Design review of the part built by this model. Coordinates are the model's own, in mm. Coordinates: 2 decimals unless noted, no trailing zeros. Answer as a JSON object with one key per item and string values.
from build123d import *

# Parameters (mm, degrees)
SWEEP1_PROFILE_R     = 13.49375
CUT_SWEEP1_PROFILE_R = 9.525


with BuildPart() as part:
    # Sweep1: sweep along a curve in space
    with BuildLine() as sweep1_path:
        Line((144.16623583, 29.78638886, -53.357198813), (145.299475263, 25.359683675, -34.863347144))
        add(Edge.make_bspline(
            [(145.299475263, 25.359683675, -34.863347144), (146.690863379, 19.924587782, -12.156649263), (145.49252871, 34.79865885, -2.165117432), (157.129656366, 36.72827895, 12.110093025)],
            knots=[0, 0, 0, 0, 1, 1, 1, 1], degree=3))
        Line((157.129656366, 36.72827895, 12.110093025), (181.072152323, 40.698324032, 41.480241636))
    # Sweep1 profile (on start of the path) → Sweep1 (sweep)
    with BuildSketch(Plane(origin=(144.16623583, 29.78638886, -53.357198813), x_dir=(0, 0.972528168, 0.232785228), z_dir=(0.059487634, -0.232372976, 0.970805862))):
        Circle(SWEEP1_PROFILE_R)
    sweep(path=sweep1_path.line)

    # Cut-Sweep1: sweep along a curve in space
    with BuildLine() as cut_sweep1_path:
        Line((144.16623583, 29.78638886, -53.357198813), (145.299475263, 25.359683675, -34.863347144))
        add(Edge.make_bspline(
            [(145.299475263, 25.359683675, -34.863347144), (146.690863379, 19.924587782, -12.156649263), (145.49252871, 34.79865885, -2.165117432), (157.129656366, 36.72827895, 12.110093025)],
            knots=[0, 0, 0, 0, 1, 1, 1, 1], degree=3))
        Line((157.129656366, 36.72827895, 12.110093025), (181.072152323, 40.698324032, 41.480241636))
    # Cut-Sweep1 profile (on start of the path) → Cut-Sweep1 (sweep, cut)
    with BuildSketch(Plane(origin=(144.16623583, 29.78638886, -53.357198813), x_dir=(0, 0.972528168, 0.232785228), z_dir=(0.059487634, -0.232372976, 0.970805862))):
        Circle(CUT_SWEEP1_PROFILE_R)
    sweep(path=cut_sweep1_path.line, mode=Mode.SUBTRACT)


solid = part.part
1) To check wall thickness, follow L1, parallel to X at y = 26, z = -14.5; L2, parallel to X at y = 30, z = -32.5; L3, parallel to Y at x = 149, z = -5.5. State the ranges of each line that lie inside material, in increasing order.
Taken from the geometry:
{"L1": "x = 132.97 to 136.96, 156.09 to 160.08", "L2": "x = 132.84 to 137.29, 153.47 to 157.92", "L3": "y = 14.91 to 19.25, 40.3 to 44.72"}
2) Insertion check: pin 1 Ø10 at (x, y) = (157, 22.5) entering from +Z; pin 2 Ø1.5 at (y, z) = (43.5, 17.5) entering from -X; pin 3 Ø1 at (x, y) = (164, 43.5) entering from -Z. Each pin has a flat end and moves straight along its axis. Give the tip position at first contact, or say it passes through.
Taken from the geometry:
{"pin 1": "stops at z = 26.97", "pin 2": "stops at x = 145.97", "pin 3": "stops at z = 1.66"}
3) Mouldability with a two-part tool opening along X and no side actions: class faces 1 (the flat face through (134.998, 26.559, -53.568)), 2 (the flat face through (173.74, 43.87, 47.03)), 3 (the cylindrical face through (176.2, 41.32, 21)) as released by +X, released by -X, zero draft, split by the parting line, or undercut.
Taken from the geometry:
{"face 1": "released by -X", "face 2": "released by +X", "face 3": "undercut"}
